Answer from the drawing. Dimensions are ordinates in mm from the lowest x, y and z of the part. A direction names the side the tool comes from. Round coordinates to 2 decimals unless told otherwise and drop trailing zeros. Loops run counter-clockwise (first coordinate to the right, second up) from the corner with the lowest first, then second, coordinate; pieces in that order, holes last. Notation, with made-up numbers: (-6.75, 1.5) - (4.25, 1.5) arc R10 cw to (4.25, 14.5) - close; hole circle Ø2 at (-21.75, 22.25). An arc over 180 degrees is marked (long way). Write item = value, one per line. Start each with the question number.
1) Section C-C, the plane y = 11 is taken. Determine the outline of the cut face in (x, z).
2) For a pull along X with two mould halves and no side action, classify the marked faces 3, 4 and 5 as released by +X, released by -X, zero draft, split by the parting line, or undercut.
3) Straight lines are drawn through the part: line 1 along Y through (x, z) = (55, 16.5); line 2 along Z through (x, y) = (32.5, 7.5); line 3 along Z through (x, y) = (49, 3.5). For each, find the intervals that lie inside material, in ascending order.
4) A tool of negligible diameter and unlimited length cuts with its end or side. For the marked faces 1 and 2, from which of +Z, -Z, +X, -X, +Y, -Y can it reach the whole face along a straight path? Write none if from no direction.
5) Section B-B, the plane z = 32.5 is taken. Determine the outline of the cut face in (x, y).
6) Given pin 1 Ø1 at (x, y) = (42.5, 10) entering from +Z; pin 2 Ø1 at (y, z) = (8.5, 39) entering from -X; pin 3 Ø8 at (x, y) = (56, 4.5) entering from -Z, each flat-ended and moving along its own axis, determine where each tip first touches the part or whether it passes through.
7) Section A-A, the plane x = 32.5 is taken. Determine the outline of the cut face in (y, z).
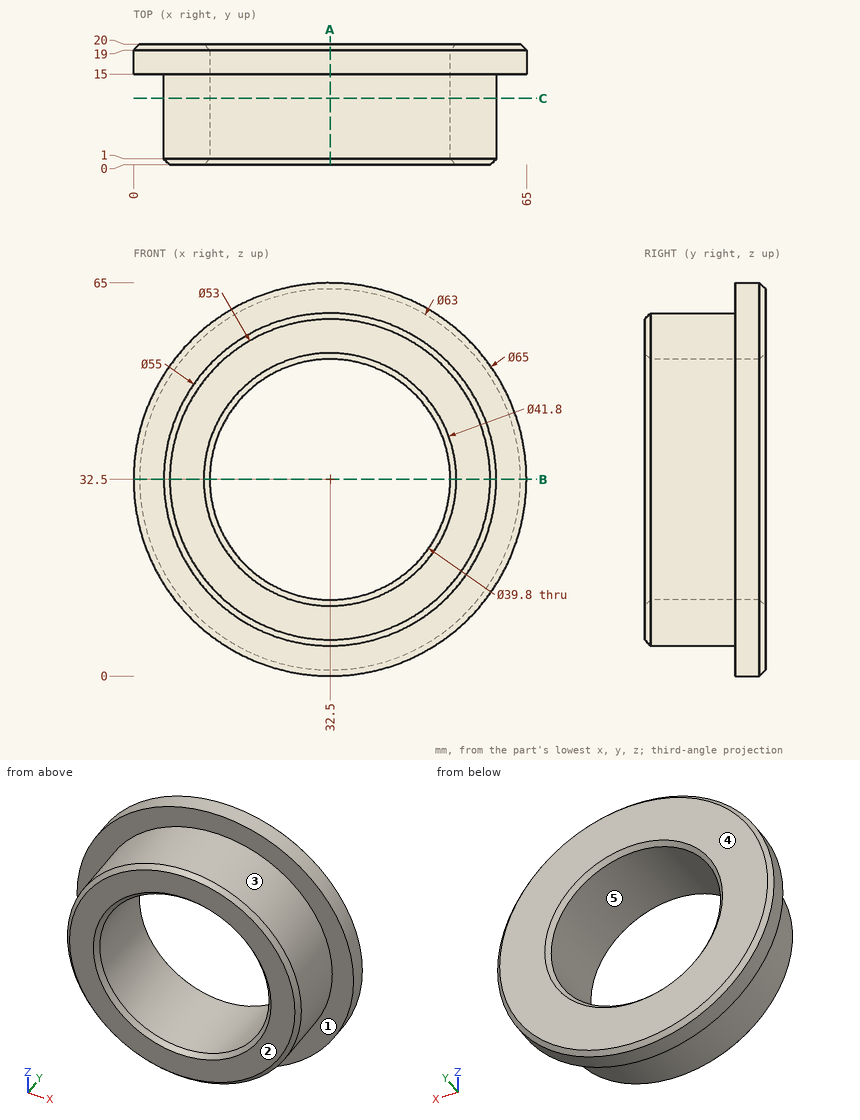
Geometry check:
q1.outline = circle Ø55 at (32.5, 32.5); hole circle Ø39.8 at (32.5, 32.5)
q2.face_3 = split by the parting line
q2.face_4 = zero draft
q2.face_5 = undercut
q3.line_1 = 15 to 20
q3.line_2 = 5 to 12.6, 52.4 to 60
q3.line_3 = 10.5 to 21.38, 43.62 to 54.5
q4.face_1 = -Y
q4.face_2 = +Z, -Z, +X, -X, -Y
q5.outline = (0, 15) - (5, 15) - (5, 1) - (6, 0) - (11.6, 0) - (12.6, 1) - (12.6, 19) - (11.6, 20) - (1, 20) - (0, 19) - close; (52.4, 1) - (53.4, 0) - (59, 0) - (60, 1) - (60, 15) - (65, 15) - (65, 19) - (64, 20) - (53.4, 20) - (52.4, 19) - close
q6.pin_1 = 58.31
q6.pin_2 = 5.66
q6.pin_3 = 13.11
q7.outline = (0, 6) - (1, 5) - (15, 5) - (15, 0) - (19, 0) - (20, 1) - (20, 11.6) - (19, 12.6) - (1, 12.6) - (0, 11.6) - close; (0, 53.4) - (1, 52.4) - (19, 52.4) - (20, 53.4) - (20, 64) - (19, 65) - (15, 65) - (15, 60) - (1, 60) - (0, 59) - close
